Geometry check sheet. Reference: the model listing, model coordinates, mm. A direction names the side the tool comes from. Round coordinates to 2 decimals unless told otherwise and drop trailing zeros. Loops run counter-clockwise (first coordinate to the right, second up) from the corner with the lowest first, then second, coordinate; pieces in that order, holes last. Notation, with made-up numbers: M -33.5,31 L 13.5,31 A33 cw 13.5,61 Z; hole C 57.5,82.25 d4. An arc over 180 degrees is marked long. Use one line per item in the form item = value. Start each with the question number.
1. Cross-section at B-B (z = -223). Record the boundary of the cut face in (x, y).
2. Go/stop test with flat-tipped pins: pin 1 (1.7 mm diameter, centred on x = 45, y = 60.5, fed in from +Z); pin 2 (5 mm diameter, centred on x = 127, z = -232.5, fed in from +Y); pin 3 (1.5 mm diameter, centred on x = 140.5, z = -69, fed in from +Y). Record where each tip stops, or that it passes through.
3. Cross-section at A-A (z = -136). Record the boundary of the cut face in (x, y).
4. Cross-section at C-C (x = 97.5). Record the boundary of the cut face in (y, z), then the cut area to 3 significant figures.
5. Draft check along Y on faces 5 (the flat face through (72.072, 49, -249)), 6 (the flat face through (125, 57, -243.84)), 7 (the flat face through (193, 11.01, -234)). Enter one of: pulls with the +Y half, pulls with the -Y half, needs draft (parallel to the pull), parting line crosses it, or undercut.
6. Material ranges on line 1 (Y direction, x = 250.95, z = -203.2); line 2 (Z direction, x = 193.04, y = 13.6); line 3 (X direction, y = 65, z = -206), recorded low to high.
7. Set-up check for faces 1 (the flat face through (5, 88.9, -141)), 2 (the flat face through (130, 16.51, -236)), 3 (the cylindrical face through (43.625, 58.85, -2.711)), 4 (the flat face through (76, 38, -248.5)): record each of +Z, -Z, +X, -X, +Y, -Y from which the full face is reachable in a straight line by a thin tool's end or side.
```python
from build123d import *

# Parameters (mm, degrees)
SKETCH1_W           = 254
SKETCH1_H           = 254
BOSS_EXTRUDE1_DEPTH = 101.6
SKETCH2_W           = 233.68
SKETCH2_H           = 233.68
CUT_EXTRUDE1_DEPTH  = 91.44
CUT_EXTRUDE10_REACH = 375.302
F_12_PIN_MOUNT_R    = 2.7999944
CUT_EXTRUDE3_DEPTH  = 5.499989
CUT_EXTRUDE5_REACH  = 375.302
CUT_EXTRUDE6_START  = -254
CUT_EXTRUDE6_DEPTH  = 10.16
SKETCH6_R           = 2.7999944
CUT_EXTRUDE7_DEPTH  = 5.499989
CUT_EXTRUDE8_START  = -248.500011
SKETCH6_2_R         = 2.7999944
CUT_EXTRUDE8_DEPTH  = 5.499989
SKETCH7_R           = 5
BOSS_EXTRUDE2_DEPTH = 6.35
CUT_EXTRUDE9_START  = 6.35
SKETCH8_R           = 2.7999944
CUT_EXTRUDE9_DEPTH  = 5.499989
CUT_EXTRUDE11_REACH = 375.302
SKETCH14_W          = 127
SKETCH14_H          = 50.8


with BuildPart() as part:
    # Sketch1 → Boss-Extrude1 (new body)
    with BuildSketch(Plane(origin=(0, 0, 0), x_dir=(1, 0, 0), z_dir=(0, 1, 0))):
        with Locations((127, 127)):
            Rectangle(SKETCH1_W, SKETCH1_H)
    extrude(amount=BOSS_EXTRUDE1_DEPTH)

    # Sketch2 → Cut-Extrude1 (cut)
    with BuildSketch(Plane(origin=(0, 101.6, 0), x_dir=(1, 0, 0), z_dir=(0, 1, 0))):
        with Locations((127, 127)):
            Rectangle(SKETCH2_W, SKETCH2_H)
    extrude(amount=-CUT_EXTRUDE1_DEPTH, mode=Mode.SUBTRACT)

    # Cut-Sweep2: sweep along a path in Sketch3
    with BuildLine(Plane(origin=(0, 101.6, 0), x_dir=(1, 0, 0), z_dir=(0, 1, 0))) as cut_sweep2_path:
        Line((6.35, 11.43), (6.35, 242.57))
        ThreePointArc((6.35, 242.57), (7.837897552, 246.162102448), (11.43, 247.65))
        Line((11.43, 247.65), (242.57, 247.65))
        ThreePointArc((242.57, 247.65), (246.162102448, 246.162102448), (247.65, 242.57))
        Line((247.65, 242.57), (247.65, 11.43))
        ThreePointArc((247.65, 11.43), (246.162102448, 7.837897552), (242.57, 6.35))
        Line((242.57, 6.35), (11.43, 6.35))
        ThreePointArc((11.43, 6.35), (7.837897552, 7.837897552), (6.35, 11.43))
    # Sketch4 → Cut-Sweep2 (sweep, cut)
    with BuildSketch(Plane.XY.offset(-15.24)):
        Polygon((4.064, 101.6), (3.272383398, 99.822), (7.141616602, 99.822), (6.35, 101.6), align=None)
    sweep(path=cut_sweep2_path.line, mode=Mode.SUBTRACT)

    # Sketch13 → Cut-Extrude10 (cut, up to next)
    with BuildSketch(Plane(origin=(254, 0, 0), x_dir=(0, 0, -1), z_dir=(1, 0, 0)), mode=Mode.PRIVATE) as cut_extrude10_sk1:
        with BuildLine():
            Line((55.735714122, 56.896), (54.2925, 56.896))
            ThreePointArc((54.2925, 56.896), (53.214869265, 56.449630735), (52.7685, 55.372))
            Line((52.7685, 55.372), (52.7685, 44.704))
            ThreePointArc((52.7685, 44.704), (53.214869265, 43.626369265), (54.2925, 43.18))
            Line((54.2925, 43.18), (55.735714122, 43.18))
            ThreePointArc((55.735714122, 43.18), (56.109218307, 43.082182673), (56.386829629, 42.813844156))
            ThreePointArc((56.386829629, 42.813844156), (58.959361214, 40.327240562), (62.4205, 39.4208))
            Line((62.4205, 39.4208), (84.1375, 39.4208))
            ThreePointArc((84.1375, 39.4208), (87.094150798, 40.069608753), (89.507465925, 41.896805195))
            ThreePointArc((89.507465925, 41.896805195), (89.767895615, 42.093984667), (90.086958651, 42.164))
            Line((90.086958651, 42.164), (92.2655, 42.164))
            ThreePointArc((92.2655, 42.164), (93.343130735, 42.610369265), (93.7895, 43.688))
            Line((93.7895, 43.688), (93.7895, 56.388))
            ThreePointArc((93.7895, 56.388), (93.343130735, 57.465630735), (92.2655, 57.912))
            Line((92.2655, 57.912), (90.086958651, 57.912))
            ThreePointArc((90.086958651, 57.912), (89.767895615, 57.982015333), (89.507465925, 58.179194805))
            ThreePointArc((89.507465925, 58.179194805), (87.094150798, 60.006391247), (84.1375, 60.6552))
            Line((84.1375, 60.6552), (62.4205, 60.6552))
            ThreePointArc((62.4205, 60.6552), (58.959361214, 59.748759438), (56.386829629, 57.262155844))
            ThreePointArc((56.386829629, 57.262155844), (56.109218307, 56.993817327), (55.735714122, 56.896))
        make_face()
    cut_extrude10_tool1 = extrude(cut_extrude10_sk1.sketch, amount=-CUT_EXTRUDE10_REACH, mode=Mode.PRIVATE) & part.part
    # Sketch13 → Cut-Extrude10 (cut, up to next)
    with BuildSketch(Plane(origin=(254, 0, 0), x_dir=(0, 0, -1), z_dir=(1, 0, 0)), mode=Mode.PRIVATE) as cut_extrude10_sk2:
        with BuildLine():
            Line((163.177714122, 56.896), (161.7345, 56.896))
            ThreePointArc((161.7345, 56.896), (160.656869265, 56.449630735), (160.2105, 55.372))
            Line((160.2105, 55.372), (160.2105, 44.704))
            ThreePointArc((160.2105, 44.704), (160.656869265, 43.626369265), (161.7345, 43.18))
            Line((161.7345, 43.18), (163.177714122, 43.18))
            ThreePointArc((163.177714122, 43.18), (163.551218307, 43.082182673), (163.828829629, 42.813844156))
            ThreePointArc((163.828829629, 42.813844156), (166.401361214, 40.327240562), (169.8625, 39.4208))
            Line((169.8625, 39.4208), (191.5795, 39.4208))
            ThreePointArc((191.5795, 39.4208), (194.536150798, 40.069608753), (196.949465925, 41.896805195))
            ThreePointArc((196.949465925, 41.896805195), (197.209895615, 42.093984667), (197.528958651, 42.164))
            Line((197.528958651, 42.164), (199.7075, 42.164))
            ThreePointArc((199.7075, 42.164), (200.785130735, 42.610369265), (201.2315, 43.688))
            Line((201.2315, 43.688), (201.2315, 56.388))
            ThreePointArc((201.2315, 56.388), (200.785130735, 57.465630735), (199.7075, 57.912))
            Line((199.7075, 57.912), (197.528958651, 57.912))
            ThreePointArc((197.528958651, 57.912), (197.209895615, 57.982015333), (196.949465925, 58.179194805))
            ThreePointArc((196.949465925, 58.179194805), (194.536150798, 60.006391247), (191.5795, 60.6552))
            Line((191.5795, 60.6552), (169.8625, 60.6552))
            ThreePointArc((169.8625, 60.6552), (166.401361214, 59.748759438), (163.828829629, 57.262155844))
            ThreePointArc((163.828829629, 57.262155844), (163.551218307, 56.993817327), (163.177714122, 56.896))
        make_face()
    cut_extrude10_tool2 = extrude(cut_extrude10_sk2.sketch, amount=-CUT_EXTRUDE10_REACH, mode=Mode.PRIVATE) & part.part
    add(cut_extrude10_tool1.solids().sort_by_distance((254, 50.038, -73.454803))[0], mode=Mode.SUBTRACT)
    add(cut_extrude10_tool2.solids().sort_by_distance((254, 50.038, -180.896803))[0], mode=Mode.SUBTRACT)

    # 12 pin mount → Cut-Extrude3 (cut)
    with BuildSketch(Plane(origin=(254, 0, 0), x_dir=(0, 0, -1), z_dir=(1, 0, 0))):
        with Locations((95.758, 61.976)):
            Circle(F_12_PIN_MOUNT_R)
        with Locations((95.758, 38.1)):
            Circle(F_12_PIN_MOUNT_R)
        with Locations((50.8, 38.1)):
            Circle(F_12_PIN_MOUNT_R)
        with Locations((50.8, 61.976)):
            Circle(F_12_PIN_MOUNT_R)
        with Locations((158.242, 61.976)):
            Circle(F_12_PIN_MOUNT_R)
        with Locations((203.2, 61.976)):
            Circle(F_12_PIN_MOUNT_R)
        with Locations((203.2, 38.1)):
            Circle(F_12_PIN_MOUNT_R)
        with Locations((158.242, 38.1)):
            Circle(F_12_PIN_MOUNT_R)
    extrude(amount=-CUT_EXTRUDE3_DEPTH, mode=Mode.SUBTRACT)

    # 4 pin connector → Cut-Extrude5 (cut, up to next)
    with BuildSketch(Plane.XY, mode=Mode.PRIVATE) as cut_extrude5_sk1:
        with BuildLine():
            Line((53.7845, 59.817), (68.2625, 59.817))
            ThreePointArc((68.2625, 59.817), (70.956576836, 58.701076836), (72.0725, 56.007))
            Line((72.0725, 56.007), (72.0725, 42.6466))
            ThreePointArc((72.0725, 42.6466), (70.956576836, 39.952523164), (68.2625, 38.8366))
            Line((68.2625, 38.8366), (53.7845, 38.8366))
            ThreePointArc((53.7845, 38.8366), (51.090423164, 39.952523164), (49.9745, 42.6466))
            Line((49.9745, 42.6466), (49.9745, 56.007))
            ThreePointArc((49.9745, 56.007), (51.090423164, 58.701076836), (53.7845, 59.817))
        make_face()
    cut_extrude5_tool1 = extrude(cut_extrude5_sk1.sketch, amount=-CUT_EXTRUDE5_REACH, mode=Mode.PRIVATE) & part.part
    add(cut_extrude5_tool1.solids().sort_by_distance((61.0235, 49.3268, 0))[0], mode=Mode.SUBTRACT)

    # Sketch5<2> → Cut-Extrude6 (cut)
    with BuildSketch(Plane.XY.offset(CUT_EXTRUDE6_START)):
        with BuildLine():
            Line((53.7845, 59.817), (68.2625, 59.817))
            ThreePointArc((68.2625, 59.817), (70.956576836, 58.701076836), (72.0725, 56.007))
            Line((72.0725, 56.007), (72.0725, 42.6466))
            ThreePointArc((72.0725, 42.6466), (70.956576836, 39.952523164), (68.2625, 38.8366))
            Line((68.2625, 38.8366), (53.7845, 38.8366))
            ThreePointArc((53.7845, 38.8366), (51.090423164, 39.952523164), (49.9745, 42.6466))
            Line((49.9745, 42.6466), (49.9745, 56.007))
            ThreePointArc((49.9745, 56.007), (51.090423164, 58.701076836), (53.7845, 59.817))
        make_face()
    extrude(amount=CUT_EXTRUDE6_DEPTH, mode=Mode.SUBTRACT)

    # Sketch6 → Cut-Extrude7 (cut)
    with BuildSketch(Plane.XY):
        with Locations((76.2, 60.5536)):
            Circle(SKETCH6_R)
        with Locations((76.2, 38.1)):
            Circle(SKETCH6_R)
        with Locations((45.847, 38.1)):
            Circle(SKETCH6_R)
        with Locations((45.847, 60.5536)):
            Circle(SKETCH6_R)
    extrude(amount=-CUT_EXTRUDE7_DEPTH, mode=Mode.SUBTRACT)

    # Sketch6<2> → Cut-Extrude8 (cut)
    with BuildSketch(Plane.XY.offset(CUT_EXTRUDE8_START)):
        with Locations((76.2, 60.5536)):
            Circle(SKETCH6_2_R)
        with Locations((76.2, 38.1)):
            Circle(SKETCH6_2_R)
        with Locations((45.847, 38.1)):
            Circle(SKETCH6_2_R)
        with Locations((45.847, 60.5536)):
            Circle(SKETCH6_2_R)
    extrude(amount=-CUT_EXTRUDE8_DEPTH, mode=Mode.SUBTRACT)

    # Sketch7 → Boss-Extrude2 (add)
    with BuildSketch(Plane(origin=(0, 10.16, 0), x_dir=(1, 0, 0), z_dir=(0, 1, 0))):
        with Locations(Location((127.38, 144.673865575, 0), (0, 0, 90))):
            Circle(SKETCH7_R)
        with Locations(Location((193.04, 144.673865575, 0), (0, 0, 90))):
            Circle(SKETCH7_R)
        with Locations(Location((193.04, 233.703865575, 0), (0, 0, 90))):
            Circle(SKETCH7_R)
        with Locations(Location((127.38, 233.703865575, 0), (0, 0, 90))):
            Circle(SKETCH7_R)
    extrude(amount=BOSS_EXTRUDE2_DEPTH)

    # Sketch8 → Cut-Extrude9 (cut)
    with BuildSketch(Plane(origin=(0, 10.16, 0), x_dir=(1, 0, 0), z_dir=(0, 1, 0)).offset(CUT_EXTRUDE9_START)):
        with Locations(Location((127.38, 233.703865575, 0), (0, 0, 270))):
            Circle(SKETCH8_R)
        with Locations(Location((193.04, 233.703865575, 0), (0, 0, 270))):
            Circle(SKETCH8_R)
        with Locations(Location((193.04, 144.673865575, 0), (0, 0, 270))):
            Circle(SKETCH8_R)
        with Locations(Location((127.38, 144.673865575, 0), (0, 0, 270))):
            Circle(SKETCH8_R)
    extrude(amount=-CUT_EXTRUDE9_DEPTH, mode=Mode.SUBTRACT)

    # Sketch14 → Cut-Extrude11 (cut, up to next)
    with BuildSketch(Plane.ZY, mode=Mode.PRIVATE) as cut_extrude11_sk1:
        with Locations((-139.7, 63.5)):
            Rectangle(SKETCH14_W, SKETCH14_H)
    cut_extrude11_tool1 = extrude(cut_extrude11_sk1.sketch, amount=-CUT_EXTRUDE11_REACH, mode=Mode.PRIVATE) & part.part
    add(cut_extrude11_tool1.solids().sort_by_distance((0, 63.5, -139.7))[0], mode=Mode.SUBTRACT)


solid = part.part
```
Reported:
q1.outline = M 0,0 L 254,0 L 254,101.6 L 249.94,101.6 L 250.73,99.82 L 246.86,99.82 L 247.65,101.6 L 243.84,101.6 L 243.84,10.16 L 10.16,10.16 L 10.16,101.6 L 6.35,101.6 L 7.14,99.82 L 3.27,99.82 L 4.06,101.6 L 0,101.6 Z
q2.pin_1 = -5.5
q2.pin_2 = 16.51
q2.pin_3 = 10.16
q3.outline = M 0,0 L 254,0 L 254,101.6 L 249.94,101.6 L 250.73,99.82 L 246.86,99.82 L 247.65,101.6 L 243.84,101.6 L 243.84,10.16 L 10.16,10.16 L 10.16,38.1 L 0,38.1 Z; M 0,88.9 L 10.16,88.9 L 10.16,101.6 L 6.35,101.6 L 7.14,99.82 L 3.27,99.82 L 4.06,101.6 L 0,101.6 Z
q4.outline = M 0,-254 L 101.6,-254 L 101.6,-249.94 L 99.82,-250.73 L 99.82,-246.86 L 101.6,-247.65 L 101.6,-243.84 L 10.16,-243.84 L 10.16,-10.16 L 101.6,-10.16 L 101.6,-6.35 L 99.82,-7.14 L 99.82,-3.27 L 101.6,-4.06 L 101.6,0 L 0,0 Z
q4.area = 4,430 mm²
q5.face_5 = undercut
q5.face_6 = needs draft
q5.face_7 = pulls with the +Y half
q6.line_1 = 0 to 35.3, 40.9 to 59.18, 64.78 to 101.6
q6.line_2 = -254 to -243.84, -238.7 to -236.5, -230.9 to -228.7, -149.67 to -147.47, -141.87 to -139.67, -10.16 to 0
q6.line_3 = 0 to 10.16, 243.84 to 254
q7.face_1 = -X
q7.face_2 = +Y
q7.face_3 = +Z
q7.face_4 = -Z
